Source: CAD feature listing. Evaluate the final solid. Frame: model axes, mm. Round coordinates to 2 decimals unless told otherwise and drop trailing zeros. Loops run counter-clockwise (first coordinate to the right, second up) from the corner with the lowest first, then second, coordinate; pieces in that order, holes last. Notation, with made-up numbers: (14, 7) -> (40, 7) arc R22 cw to (40, 23) -> close; hole circle Ø8 at (-6, -9.75). An arc over 180 degrees is marked (long way). Write item = value, one per line.
from build123d import *

# Parameters (mm, degrees)
F1_DEPTH = 6.35
F3_D     = 7
F4_D     = 15


with BuildPart() as f1:
    # F0 (on Front) → F1 (new body)
    with BuildSketch(Plane.XZ):
        with BuildLine():
            Line((-79.2936884003, 62.5334825695), (-109.2936884003, 62.5334825695))
            Line((-109.2936884003, 62.5334825695), (-109.2936884003, -62.4665174305))
            Line((-109.2936884003, -62.4665174305), (140.7063115997, -62.4665174305))
            Line((140.7063115997, -62.4665174305), (140.7063115997, -32.4665174305))
            ThreePointArc((140.7063115997, -32.4665174305), (134.8484472234, -18.3243818068), (120.7063115997, -12.4665174305))
            Line((120.7063115997, -12.4665174305), (-39.2936884003, -12.4665174305))
            ThreePointArc((-39.2936884003, -12.4665174305), (-53.435824024, -6.6086530543), (-59.2936884003, 7.5334825695))
            Line((-59.2936884003, 7.5334825695), (-59.2936884003, 42.5334825695))
            ThreePointArc((-59.2936884003, 42.5334825695), (-65.1515527766, 56.6756181932), (-79.2936884003, 62.5334825695))
        make_face()
    extrude(amount=F1_DEPTH)

    # F3 (through all)
    with Locations(Plane(origin=(0, 0, 0), x_dir=(1, 0, 0), z_dir=(0, 1, 0))):
        with Locations((-94.2936884003, -49.5334825695), (-94.2936884003, 47.4665174305)):
            Hole(F3_D / 2)

    # F4 (through all)
    with Locations(Plane(origin=(0, 0, 0), x_dir=(1, 0, 0), z_dir=(0, 1, 0))):
        with Locations((100.7063115997, 37.8665174305)):
            Hole(F4_D / 2)


solid = f1.part
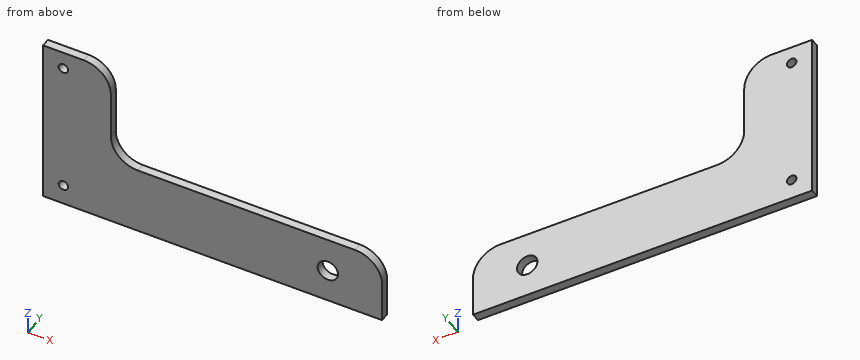
1. Section query C-C (z = 23.5). Return the cut outline in (x, y).
Evaluation:
outline = (-109.29, -6.35) -> (-59.29, -6.35) -> (-59.29, 0) -> (-109.29, 0) -> close
2. Line query: probe 1 along X at (y, z) = (-1.25, 7.5); probe 2 along Z at (x, y) = (-78, -2.75); probe 3 along X at (y, z) = (-0.75, -41.5). Output: solid intervals per line, ascending. Write a range as from..to.
Evaluation:
probe_1 = -109.29..-59.29
probe_2 = -62.47..62.49
probe_3 = -109.29..94.15, 107.27..140.71
3. Section query B-B (x = 22.5). Return the cut outline in (y, z).
Evaluation:
outline = (-6.35, -62.47) -> (0, -62.47) -> (0, -12.47) -> (-6.35, -12.47) -> close
4. Contact query for flat-ended pins moving along their axis: pin 1 Ø1 at (y, z) = (-5.5, 45) entering from +X; pin 2 Ø5.5 at (x, z) = (-94.29, 49.53) entering from -Y. Output: stop coordinate, or through.
Evaluation:
pin_1 = -59.39
pin_2 = through
5. Section query A-A (y = -3.75). Return the cut outline in (x, z).
Evaluation:
outline = (-109.29, -62.47) -> (140.71, -62.47) -> (140.71, -32.47) arc R20 ccw to (120.71, -12.47) -> (-39.29, -12.47) arc R20 cw to (-59.29, 7.53) -> (-59.29, 42.53) arc R20 ccw to (-79.29, 62.53) -> (-109.29, 62.53) -> close; hole circle Ø7 at (-94.29, -47.47); hole circle Ø7 at (-94.29, 49.53); hole circle Ø15 at (100.71, -37.87)
